```python
from build123d import *

# Parameters (mm, degrees)
F1_DEPTH = 19
F4_DEPTH = 28
F9_DEPTH = 9.5


with BuildPart() as f1:
    # F0 (on Front) → F1 (new body)
    with BuildSketch(Plane.XZ):
        Polygon((-38, 0), (0, 0), (0, 55), (-38, 60), align=None)
    extrude(amount=-F1_DEPTH)

    # F3 (on 3pt) → F4 (cut, symmetric)
    with BuildSketch(Plane(origin=(-7.1136827774, 0, 0.9360108918), x_dir=(0, -1, 0), z_dir=(-0.9914542955, 0, 0.1304545126))):
        with BuildLine():
            Line((-1.5, 54.5299862548), (-17.5, 54.5299862548))
            ThreePointArc((-17.5, 54.5299862548), (-9.5, 46.5299862548), (-1.5, 54.5299862548))
        make_face()
    extrude(amount=F4_DEPTH, both=True, mode=Mode.SUBTRACT)

    # F6 (on offset) → F7 (revolve, cut)
    with BuildSketch(Plane(origin=(-34.8744030526, 0, 4.5887372438), x_dir=(0, 1, 0), z_dir=(0.9914542955, 0, -0.1304545126))):
        with BuildLine():
            ThreePointArc((9.5, 46.5299862548), (15.1568542495, 48.8731320053), (17.5, 54.5299862548))
            Line((17.5, 54.5299862548), (9.5, 54.5299862548))
            Line((9.5, 54.5299862548), (9.5, 46.5299862548))
        make_face()
    revolve(axis=Axis((-28.2825383255, 9.5, 54.6869091698), (0.1304545126, 0, 0.9914542955)), mode=Mode.SUBTRACT)

    # F8 (on Front) → F9 (cut)
    with BuildSketch(Plane.XZ):
        with BuildLine():
            ThreePointArc((-35.6923546395, 59.6963624526), (-28.8043563758, 50.7210919877), (-19.8290859109, 57.6090902514))
            Line((-19.8290859109, 57.6090902514), (-35.6923546395, 59.6963624526))
        make_face()
    extrude(amount=-F9_DEPTH, mode=Mode.SUBTRACT)


solid = f1.part
```
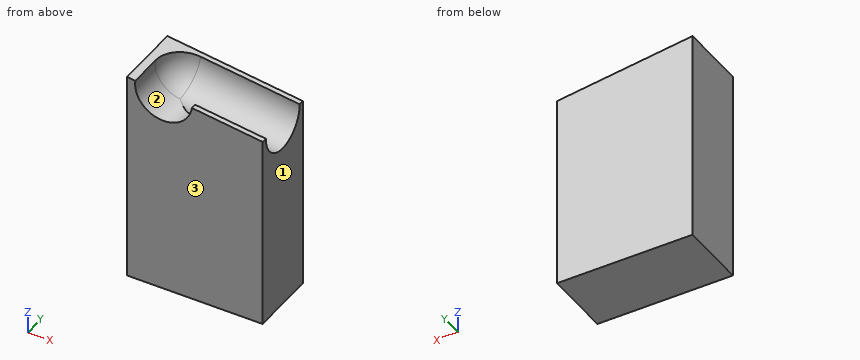
Check sheet for the modelled part. Datum: model origin and axes. Units: mm. Face numbers are marked on the shaded views. Round coordinates to 2 decimals unless told otherwise and drop trailing zeros. Write each loop counter-clockwise with the first axis right and the second up, starting at its lowest first coordinate (ties: lowest second). Pieces come first, ordered by that corner, then holes. Notation, with made-up numbers: (67.5, 55) -> (105.5, 55) arc R26 cw to (105.5, 79) -> close; hole circle Ø8 at (43, -14). An arc over 180 degrees is marked (long way). One line per question, with ' | ' between items. Start each with the question number.
1. Scan lines: line 1 along Z through (x, y) = (-15, 5); line 2 along Z through (x, y) = (-13.5, 11.75); line 3 along Y through (x, z) = (-24, 54.5). Record each from-to range of solid material in increasing order. Write a range as from..to.
2. Sectioned sample at A-A, the plane y = 7. Record the cut outline in (x, z), then the cut area to 3 significant figures.
3. Depth check by flat-ended pin: pin 1 (1 mm diameter, centred on y = 4.5, z = 53, fed in from +X); pin 2 (10 mm diameter, centred on x = -21, y = 7.5, fed in from +Z); pin 3 (1 mm diameter, centred on x = -24.5, y = 12.5, fed in from +Z). Enter the tip coordinate at first touch or a pass-through.
4. Sectioned sample at B-B, the plane x = -30. Record the cut outline in (y, z).
5. Release check for a two-part mould opening along X. For the marked faces 1, 2 and 3 record: +X half, -X half, draft (parallel to the pull), parting line (faces both ways), or undercut.
Taken from the geometry:
1) line 1: z = 0..50.3 | line 2: z = 0..49.03 | line 3: y = 16.63..19
2) outline: (-38, 0) -> (0, 0) -> (0, 47.34) -> (-26.27, 50.79) arc R8 cw to (-35.69, 59.7) -> (-38, 60) -> close | area: 1,920 mm^2
3) pin 1: stops at x = -32.87 | pin 2: stops at z = 53.88 | pin 3: stops at z = 50.98
4) outline: (0, 0) -> (19, 0) -> (19, 58.95) -> (17.17, 58.95) arc R7.68 cw to (9.5, 50.97) -> (0, 50.97) -> close
5) face 1: +X half | face 2: undercut | face 3: draft
